```python
from build123d import *

# Parameters (mm, degrees)
SKETCH1_W           = 109
SKETCH1_H           = 133
BOSS_EXTRUDE1_DEPTH = 62
SKETCH3_W           = 3
SKETCH3_H           = 77
CUT_EXTRUDE2_DEPTH  = 109
SKETCH4_W           = 12
SKETCH4_H           = 127
CUT_EXTRUDE3_DEPTH  = 109
SKETCH5_W           = 45
SKETCH5_H           = 65
CUT_EXTRUDE4_DEPTH  = 107
SKETCH6_W           = 105
SKETCH6_H           = 10
CUT_EXTRUDE5_DEPTH  = 45
SKETCH7_W           = 105
SKETCH7_H           = 50
CUT_EXTRUDE6_DEPTH  = 45
SKETCH9_W           = 105
SKETCH9_H           = 32
CUT_EXTRUDE7_DEPTH  = 45
SKETCH11_W          = 3
SKETCH11_H          = 10
CUT_EXTRUDE9_DEPTH  = 192
SKETCH10_W          = 65
SKETCH10_H          = 30
CUT_EXTRUDE10_DEPTH = 10
SKETCH14_W          = 2
SKETCH14_H          = 45
BOSS_EXTRUDE2_DEPTH = 2.5


with BuildPart() as part:
    # Sketch1 → Boss-Extrude1 (new body)
    with BuildSketch(Plane.XY):
        Rectangle(SKETCH1_W, SKETCH1_H)
    extrude(amount=BOSS_EXTRUDE1_DEPTH)

    # Sketch3 → Cut-Extrude2 (cut)
    with BuildSketch(Plane.ZY.offset(54.5)):
        with Locations((60.5, 0)):
            Rectangle(SKETCH3_W, SKETCH3_H)
    extrude(amount=-CUT_EXTRUDE2_DEPTH, mode=Mode.SUBTRACT)

    # Sketch4 → Cut-Extrude3 (cut)
    with BuildSketch(Plane.ZY.offset(54.5)):
        with Locations((53, 0)):
            Rectangle(SKETCH4_W, SKETCH4_H)
    extrude(amount=-CUT_EXTRUDE3_DEPTH, mode=Mode.SUBTRACT)

    # Sketch5 → Cut-Extrude4 (cut)
    with BuildSketch(Plane.ZY.offset(54.5)):
        with Locations((24.5, -31)):
            Rectangle(SKETCH5_W, SKETCH5_H)
    extrude(amount=-CUT_EXTRUDE4_DEPTH, mode=Mode.SUBTRACT)

    # Sketch6 → Cut-Extrude5 (cut)
    with BuildSketch(Plane.XY.offset(47)):
        with Locations((0, 6.5)):
            Rectangle(SKETCH6_W, SKETCH6_H)
    extrude(amount=-CUT_EXTRUDE5_DEPTH, mode=Mode.SUBTRACT)

    # Sketch7 → Cut-Extrude6 (cut)
    with BuildSketch(Plane.XY.offset(47)):
        with Locations((0, 38.5)):
            Rectangle(SKETCH7_W, SKETCH7_H)
    extrude(amount=-CUT_EXTRUDE6_DEPTH, mode=Mode.SUBTRACT)

    # Sketch9 → Cut-Extrude7 (cut)
    with BuildSketch(Plane(origin=(0, 0, 0), x_dir=(-1, 0, 0), z_dir=(0, 0, -1))):
        with Locations((0, 38.5)):
            Rectangle(SKETCH9_W, SKETCH9_H)
    extrude(amount=-CUT_EXTRUDE7_DEPTH, mode=Mode.SUBTRACT)

    # Sketch11 → Cut-Extrude9 (cut)
    with BuildSketch(Plane.ZY.offset(54.5)):
        with Locations((60.5, 43.5)):
            Rectangle(SKETCH11_W, SKETCH11_H)
        with Locations((60.5, -43.5)):
            Rectangle(SKETCH11_W, SKETCH11_H)
    extrude(amount=-CUT_EXTRUDE9_DEPTH, mode=Mode.SUBTRACT)

    # Sketch10 → Cut-Extrude10 (cut)
    with BuildSketch(Plane.XZ.offset(66.5)):
        with Locations((20, 26.022609269)):
            Rectangle(SKETCH10_W, SKETCH10_H)
    extrude(amount=-CUT_EXTRUDE10_DEPTH, mode=Mode.SUBTRACT)

    # Sketch14 → Boss-Extrude2 (add)
    with BuildSketch(Plane.XZ.offset(-1.5)):
        with Locations((-53.5, 24.5)):
            Rectangle(SKETCH14_W, SKETCH14_H)
    extrude(amount=BOSS_EXTRUDE2_DEPTH)


solid = part.part
```
Here's how the part is built. I have some questions about the finished solid (model axes, mm). A direction names the side the tool comes from. Round coordinates to 2 decimals unless told otherwise and drop trailing zeros. Write each loop counter-clockwise with the first axis right and the second up, starting at its lowest first coordinate (ties: lowest second). Pieces come first, ordered by that corner, then holes. Notation, with made-up numbers: M -9,-34.5 L 7,-34.5 A9 cw 7,-27.5 Z; hole C -22,-18 d8. An arc over 180 degrees is marked long. Answer as CSV lines item,"result". Start each with the question number.
1. Thinking about a two-plate mould opening in X: for faces 6 (the flat face through (-54.5, 30, 24)), 7 (the flat face through (-1, -48.5, 60)), 8 (the flat face through (20, -65, 41.023)), 9 (the flat face through (54.5, -1, 24)), which applies, released by +X, released by -X, zero draft, split by the parting line, or undercut?
2. Suppose I cut it at C-C on z = 53.5. Write out the boundary of the cut face in (x, y).
3. I'm going to push flat-ended pins straight in: pin 1 Ø8 at (x, y) = (37, -5) entering from +Z; pin 2 Ø2 at (x, z) = (34.5, 13) entering from -Y. Where does each tip first touch, or does it pass through?
4. I need wall thicknesses on probe 1 along Y at (x, z) = (-26.5, 46.5); probe 2 along Y at (x, z) = (39, 14); probe 3 along X at (y, z) = (40, 17). Which ranges of each line are inside material? Lowest first, please.
5. Suppose I cut it at D-D on x = 9.5. Write out the boundary of the cut face in (y, z).
6. Suppose I cut it at A-A on z = 38. Write out the boundary of the cut face in (x, y), then the cut area to 3 significant figures.
7. On a 3-axis mill with a long thin cutter (end or side, diameter ignored), from which of +Z, -Z, +X, -X, +Y, -Y can I reach the whole of each face in a straight line? I mean faces 1 (the flat face through (-13, -63.5, 30)), 2 (the flat face through (-1, 11.5, 25)), 3 (the flat face through (-1, 59, 2)), 4 (the flat face through (-12.5, -65, 26)), 5 (the flat face through (-53, 29, 47)). Say none if no direction works.
8. Suppose I cut it at B-B on y = 50.5. Write out the boundary of the cut face in (x, z), then the cut area to 3 significant figures.
Check result:
1,face 6,"released by -X"
1,face 7,"zero draft"
1,face 8,"undercut"
1,face 9,"released by +X"
2,outline,"M -54.5,-66.5 L 54.5,-66.5 L 54.5,-63.5 L -54.5,-63.5 Z; M -54.5,63.5 L 54.5,63.5 L 54.5,66.5 L -54.5,66.5 Z"
3,pin 1,"stops at z = 2"
3,pin 2,"stops at y = 11.5"
4,probe 1,"y = -66.5 to -63.5, 11.5 to 13.5, 63.5 to 66.5"
4,probe 2,"y = 11.5 to 13.5, 63.5 to 66.5"
4,probe 3,"x = -54.5 to -52.5, 52.5 to 54.5"
5,outline,"M -66.5,0 L 22.5,0 L 22.5,2 L 13.5,2 L 13.5,47 L 11.5,47 L 11.5,2 L -63.5,2 L -63.5,11.02 L -66.5,11.02 Z; M -66.5,41.02 L -63.5,41.02 L -63.5,59 L -48.5,59 L -48.5,62 L -66.5,62 Z; M 48.5,59 L 63.5,59 L 63.5,2 L 54.5,2 L 54.5,0 L 66.5,0 L 66.5,62 L 48.5,62 Z"
6,outline,"M -54.5,-66.5 L -12.5,-66.5 L -12.5,-63.5 L -54.5,-63.5 Z; M -54.5,-1 L -52.5,-1 L -52.5,11.5 L 52.5,11.5 L 52.5,-66.5 L 54.5,-66.5 L 54.5,66.5 L -54.5,66.5 Z; hole M -52.5,13.5 L 52.5,13.5 L 52.5,63.5 L -52.5,63.5 Z"
6,area,"1,050 mm2"
7,face 1,"-X"
7,face 2,"+Z"
7,face 3,"none"
7,face 4,"-Y"
7,face 5,"+X, -X"
8,outline,"M -54.5,0 L -52.5,0 L -52.5,47 L -54.5,47 Z; M -54.5,59 L 54.5,59 L 54.5,62 L -54.5,62 Z; M 52.5,0 L 54.5,0 L 54.5,47 L 52.5,47 Z"
8,area,"515 mm2"
